from build123d import *

# Parameters (mm, degrees)
BOSS_EXTRUDE1_DEPTH = 1.5875
FILLET1_R           = 1
SKETCH2_R           = 0.45
CUT_EXTRUDE1_DEPTH  = 71.728496069
CUT_EXTRUDE2_DEPTH  = 9.8806
FILLET2_R           = 1
SKETCH4_W           = 6.5
SKETCH4_H           = 6.5
BOSS_EXTRUDE2_DEPTH = 0.01
SKETCH5_OUTSIDE_W   = 130.286
SKETCH5_OUTSIDE_H   = 130.286
SKETCH5_OUTSIDE_W_2 = 99
SKETCH5_OUTSIDE_H_2 = 100
CUT_EXTRUDE3_DEPTH  = 71.728721226


with BuildPart() as part:
    # Sketch1 → Boss-Extrude1 (new body)
    with BuildSketch(Plane.XY):
        Polygon((40, 50), (-40, 50), (-40, 48), (-48, 48), (-48, 40), (-50, 40), (-50, -37.864895224), (-50, -40), (-48, -40), (-48, -48), (-40, -48), (-40, -50), (-37.864895224, -50), (40, -50), (40, -48), (48, -48), (48, -40), (50, -40), (50, 40), (48, 40), (48, 48), (40, 48), align=None)
    extrude(amount=BOSS_EXTRUDE1_DEPTH)

    # Fillet1
    fillet1_edges = [part.edges().sort_by_distance(p)[0] for p in [
        (-48, -40, 0.79375),
        (-48, 40, 0.79375),
        (-40, 48, 0.79375),
        (40, 48, 0.79375),
        (48, 40, 0.79375),
        (48, -40, 0.79375),
        (40, -48, 0.79375),
        (-40, -48, 0.79375),
    ]]
    fillet(fillet1_edges, radius=FILLET1_R)

    # Sketch2 → Cut-Extrude1 (cut, through all)
    with BuildSketch(Plane.XY.offset(1.5875)):
        with Locations((-35, 43.55)):
            Circle(SKETCH2_R)
        with Locations((-33, 43.55)):
            Circle(SKETCH2_R)
        with Locations((-31, 43.55)):
            Circle(SKETCH2_R)
        with Locations((-29, 43.55)):
            Circle(SKETCH2_R)
        with Locations((-27, 43.55)):
            Circle(SKETCH2_R)
        with Locations((-25, 43.55)):
            Circle(SKETCH2_R)
        with Locations((-23, 43.55)):
            Circle(SKETCH2_R)
        with Locations((-21, 43.55)):
            Circle(SKETCH2_R)
        with Locations((-19, 43.55)):
            Circle(SKETCH2_R)
        with Locations((-17, 43.55)):
            Circle(SKETCH2_R)
        with Locations((-15, 43.55)):
            Circle(SKETCH2_R)
        with Locations((-13, 43.55)):
            Circle(SKETCH2_R)
        with Locations((-11, 43.55)):
            Circle(SKETCH2_R)
        with Locations((-9, 43.55)):
            Circle(SKETCH2_R)
        with Locations((-7, 43.55)):
            Circle(SKETCH2_R)
        with Locations((-5, 43.55)):
            Circle(SKETCH2_R)
        with Locations((-3, 43.55)):
            Circle(SKETCH2_R)
        with Locations((-1, 43.55)):
            Circle(SKETCH2_R)
        with Locations((1, 43.55)):
            Circle(SKETCH2_R)
        with Locations((3, 43.55)):
            Circle(SKETCH2_R)
        with Locations((5, 43.55)):
            Circle(SKETCH2_R)
        with Locations((7, 43.55)):
            Circle(SKETCH2_R)
        with Locations((-33, 41.55)):
            Circle(SKETCH2_R)
        with Locations((-31, 41.55)):
            Circle(SKETCH2_R)
        with Locations((-29, 41.55)):
            Circle(SKETCH2_R)
        with Locations((-27, 41.55)):
            Circle(SKETCH2_R)
        with Locations((-25, 41.55)):
            Circle(SKETCH2_R)
        with Locations((-23, 41.55)):
            Circle(SKETCH2_R)
        with Locations((-21, 41.55)):
            Circle(SKETCH2_R)
        with Locations((-19, 41.55)):
            Circle(SKETCH2_R)
        with Locations((-17, 41.55)):
            Circle(SKETCH2_R)
        with Locations((-15, 41.55)):
            Circle(SKETCH2_R)
        with Locations((-13, 41.55)):
            Circle(SKETCH2_R)
        with Locations((-11, 41.55)):
            Circle(SKETCH2_R)
        with Locations((-9, 41.55)):
            Circle(SKETCH2_R)
        with Locations((-7, 41.55)):
            Circle(SKETCH2_R)
        with Locations((-5, 41.55)):
            Circle(SKETCH2_R)
        with Locations((-3, 41.55)):
            Circle(SKETCH2_R)
        with Locations((-1, 41.55)):
            Circle(SKETCH2_R)
        with Locations((1, 41.55)):
            Circle(SKETCH2_R)
        with Locations((3, 41.55)):
            Circle(SKETCH2_R)
        with Locations((5, 41.55)):
            Circle(SKETCH2_R)
        with Locations((7, 41.55)):
            Circle(SKETCH2_R)
        with Locations((-35, 41.55)):
            Circle(SKETCH2_R)
    extrude(amount=-CUT_EXTRUDE1_DEPTH, mode=Mode.SUBTRACT)

    # Sketch3 → Cut-Extrude2 (cut)
    with BuildSketch(Plane(origin=(0, 50, 0), x_dir=(1, 0, 0), z_dir=(0, 1, 0))):
        Polygon((10.7, 0), (19.7, 0), (27.1, 0), (27.1, -1.5875), (19.7, -1.5875), (10.7, -1.5875), align=None)
    extrude(amount=-CUT_EXTRUDE2_DEPTH, mode=Mode.SUBTRACT)

    # Fillet2
    fillet2_edges = [part.edges().sort_by_distance(p)[0] for p in [
        (10.7, 40.1194, 0.79375),
        (27.1, 40.1194, 0.79375),
    ]]
    fillet(fillet2_edges, radius=FILLET2_R)

    # Sketch4 → Boss-Extrude2 (add)
    with BuildSketch(Plane.XY.offset(1.5875)):
        with Locations((-44.75, 44.75)):
            Rectangle(SKETCH4_W, SKETCH4_H)
        with Locations((-44.75, -44.75)):
            Rectangle(SKETCH4_W, SKETCH4_H)
        with Locations((44.75, -44.75)):
            Rectangle(SKETCH4_W, SKETCH4_H)
        with Locations((44.75, 44.75)):
            Rectangle(SKETCH4_W, SKETCH4_H)
    extrude(amount=BOSS_EXTRUDE2_DEPTH)

    # Sketch5 outside → Cut-Extrude3 (cut, through all)
    with BuildSketch(Plane(origin=(0, 0, 0), x_dir=(-1, 0, 0), z_dir=(0, 0, -1))):
        Rectangle(SKETCH5_OUTSIDE_W, SKETCH5_OUTSIDE_H)
        Rectangle(SKETCH5_OUTSIDE_W_2, SKETCH5_OUTSIDE_H_2, mode=Mode.SUBTRACT)
    extrude(amount=-CUT_EXTRUDE3_DEPTH, mode=Mode.SUBTRACT)


solid = part.part
Could you check a few things on this model? Use its own coordinates, in mm. Give positions to 0.01 mm unless a question says otherwise; leave off trailing zeros. Return JSON: item names as keys, results as strings. Group by question number.
Q1. Will these pins go through, and if not, where does the flat tip stop? pin 1 Ø8 at (x, y) = (-36, 1) entering from -Z; pin 2 Ø0.8 at (y, z) = (43.5, 0.5) entering from +X; pin 3 Ø4 at (x, y) = (0.5, 26) entering from +Z; pin 4 Ø0.8 at (y, z) = (49.5, 0.5) entering from +X.
Q2. Please list where these lines run through material, in increasing order: line 1 along Y through (x, z) = (-13, 0.7); line 2 along Z through (x, y) = (-4, -41); line 3 along Y through (x, z) = (43, 0.6). Write a range as [from, to].
Q3. Suppose I cut it at A-A, the plane z = 1.15. State how many separate pieces and enclosed holes the cut face has, and give its area (3 significant figures).
Resolved:
{
 "1": {"pin 1": "stops at z = 0", "pin 2": "stops at x = 48", "pin 3": "stops at z = 1.59", "pin 4": "stops at x = 40"},
 "2": {"line 1": "y = [-50, 41.1], [42, 43.1], [44, 50]", "line 2": "z = [0, 1.59]", "line 3": "y = [-48, 48]"},
 "3": {"separate pieces": "1", "enclosed holes": "44", "area": "9,590 mm2"}
}
